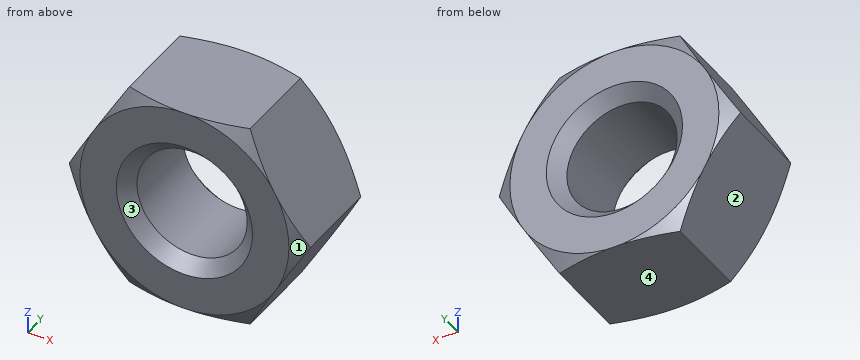
from build123d import *

# Parameters (mm, degrees)
EXTRUDE_1_DEPTH     = 8
SKETCH_2_OUTSIDE_W  = 53.488
SKETCH_2_OUTSIDE_H  = 50.996
SKETCH_2_OUTSIDE_R  = 8.054036255
CUT_EXTRUDE_2_DEPTH = 8
CUT_EXTRUDE_2_DRAFT = -60
SKETCH_3_OUTSIDE_W  = 53.488
SKETCH_3_OUTSIDE_H  = 50.996
SKETCH_3_OUTSIDE_R  = 8.054036255
CUT_EXTRUDE_3_DEPTH = 8
CUT_EXTRUDE_3_DRAFT = -60
SKETCH_4_R          = 4.25
CUT_EXTRUDE_4_DEPTH = 15.675063884
CHAMFER_1_SIZE      = 1


with BuildPart() as part:
    # Эскиз1 → Бобышка-Вытянуть1 (new body)
    with BuildSketch(Plane(origin=(0, 0, 0), x_dir=(1, 0, 0), z_dir=(0, 1, 0))):
        Polygon((9.3, 0), (4.65, 8.054036255), (-4.65, 8.054036255), (-9.3, 0), (-4.65, -8.054036255), (4.65, -8.054036255), align=None)
    extrude(amount=EXTRUDE_1_DEPTH)


with BuildPart() as cut_extrude_2_tool:
    # Эскиз2 outside → Вырез-Вытянуть2 (with draft: the straight prism first)
    with BuildSketch(Plane(origin=(0, 8, 0), x_dir=(1, 0, 0), z_dir=(0, 1, 0))):
        Rectangle(SKETCH_2_OUTSIDE_W, SKETCH_2_OUTSIDE_H)
        Circle(SKETCH_2_OUTSIDE_R, mode=Mode.SUBTRACT)
    extrude(amount=-CUT_EXTRUDE_2_DEPTH)
    # Вырез-Вытянуть2: the draft: its side faces are tilted about the plane it starts from
    cut_extrude_2_sides = [cut_extrude_2_tool.faces().sort_by_distance(p)[0] for p in [
        (0, 4, 25.498),
        (26.744, 4, 0),
        (0, 4, -25.498),
        (-26.744, 4, 0),
        (-8.054036255, 4, 0),
    ]]
    draft(cut_extrude_2_sides, Plane(origin=(0, 8, 0), x_dir=(1, 0, 0), z_dir=(0, 1, 0)), CUT_EXTRUDE_2_DRAFT)


with BuildPart() as part_1:
    add(part.part)

    # Вырез-Вытянуть2: cut by cut_extrude_2_tool
    add(cut_extrude_2_tool.part, mode=Mode.SUBTRACT)


with BuildPart() as cut_extrude_3_tool:
    # Эскиз3 outside → Вырез-Вытянуть3 (with draft: the straight prism first)
    with BuildSketch(Plane.XZ):
        Rectangle(SKETCH_3_OUTSIDE_W, SKETCH_3_OUTSIDE_H)
        Circle(SKETCH_3_OUTSIDE_R, mode=Mode.SUBTRACT)
    extrude(amount=-CUT_EXTRUDE_3_DEPTH)
    # Вырез-Вытянуть3: the draft: its side faces are tilted about the plane it starts from
    cut_extrude_3_sides = [cut_extrude_3_tool.faces().sort_by_distance(p)[0] for p in [
        (0, 4, -25.498),
        (26.744, 4, 0),
        (0, 4, 25.498),
        (-26.744, 4, 0),
        (-8.054036255, 4, 0),
    ]]
    draft(cut_extrude_3_sides, Plane.XZ, CUT_EXTRUDE_3_DRAFT)


with BuildPart() as part_2:
    add(part_1.part)

    # Вырез-Вытянуть3: cut by cut_extrude_3_tool
    add(cut_extrude_3_tool.part, mode=Mode.SUBTRACT)

    # Эскиз4 → Вырез-Вытянуть4 (cut, through all)
    with BuildSketch(Plane.XZ):
        with Locations(Location((0, 0, 0), (0, 0, 270))):
            Circle(SKETCH_4_R)
    extrude(amount=-CUT_EXTRUDE_4_DEPTH, mode=Mode.SUBTRACT)

    # Фаска1
    chamfer_1_edges = [part_2.edges().sort_by_distance(p)[0] for p in [
        (0, 8, 4.25),
        (0, 0, 4.25),
    ]]
    chamfer(chamfer_1_edges, length=CHAMFER_1_SIZE)


solid = part_2.part
The listing builds one solid part. Answer for the finished solid, in the listing's coordinates (mm). Face numbers are marked on the shaded views. Round coordinates to 2 decimals unless told otherwise and drop trailing zeros. Loops run counter-clockwise (first coordinate to the right, second up) from the corner with the lowest first, then second, coordinate; pieces in that order, holes last. Notation, with made-up numbers: M 82,40 L 121,40 A23 ccw 121,79 Z; hole C 17,63 d3. An arc over 180 degrees is marked long. Write each question's results on one line, items separated by ' | '. Start each with the question number.
1) Find section A-A on y = 6. Write down the section's boundary in (x, z), plus the area to 3 significant figures.
2) Straight lines are drawn through the part: probe 1 along Z at (x, y) = (3, 1.75); probe 2 along X at (y, z) = (7.5, -3); probe 3 along Z at (x, y) = (-0.5, 7.25). For each, find the intervals that lie inside material, in ascending order.
3) Each of these flat-tipped pins is pushed along its axis until it touches: pin 1 (1 mm diameter, centred on y = 6, z = -3.5, fed in from +X); pin 2 (1 mm diameter, centred on x = -3, z = -6, fed in from -Y); pin 3 (2 mm diameter, centred on y = 1.5, z = -6.5, fed in from +X); pin 4 (3 mm diameter, centred on y = 2.5, z = -1, fed in from -X). Where does it stop, or does it pass through?
4) Determine the mould class of the marked faces 1, 2, 3 and 4 for opening direction X: pulls with the +X half, pulls with the -X half, needs draft (parallel to the pull), parting line crosses it, or undercut.
Final values:
1) outline: M -9.3,0 L -4.65,-8.05 L 4.65,-8.05 L 9.3,0 L 4.65,8.05 L -4.65,8.05 Z; hole C 0,0 d8.5 | area: 168 mm²
2) probe 1: -8.05 to -3.01, 3.01 to 8.05 | probe 2: -7.57 to -3.68, 3.68 to 7.57 | probe 3: -8.05 to -4.47, 4.47 to 8.05
3) pin 1: x = 7.57 | pin 2: y = 0 | pin 3: x = 6.12 | pin 4: x = -9.3
4) face 1: pulls with the +X half | face 2: pulls with the -X half | face 3: undercut | face 4: needs draft
